Read the model definition and answer for the solid it produces. Units are mm, in the model's axes. A direction names the side the tool comes from. Coordinates: 2 decimals unless noted, no trailing zeros. Loops run counter-clockwise (first coordinate to the right, second up) from the corner with the lowest first, then second, coordinate; pieces in that order, holes last.
from build123d import *

# Parameters (mm, degrees)
F1_DEPTH = 7.5
F2_R     = 7.49999
F3_R     = 5
F4_DEPTH = 35.001
F5_R     = 5
F6_DEPTH = 27.501


# Not quite as in the source:
# - a fillet or chamfer is up to 0.001 mm smaller than in the source, because OpenCascade refuses the exact size


with BuildPart() as f1:
    # F0 (on Front) → F1 (new body, symmetric)
    with BuildSketch(Plane.XZ):
        with BuildLine():
            Line((7.5, 25), (-7.5, 25))
            Line((-7.5, 25), (-7.5, 20))
            Line((-7.5, 20), (7.5, 20))
            ThreePointArc((7.5, 20), (12.8033008589, 17.8033008589), (15, 12.5))
            Line((15, 12.5), (15, -10))
            Line((15, -10), (20, -10))
            Line((20, -10), (20, 12.5))
            ThreePointArc((20, 12.5), (16.3388347648, 21.3388347648), (7.5, 25))
        make_face()
    extrude(amount=F1_DEPTH, both=True)

    # F2 (radius 7.5 in the source; OpenCascade refuses exactly that, so slightly less here)
    f2_edges = [f1.edges().sort_by_distance(p)[0] for p in [
        (-7.5, -7.5, 22.5),
        (-7.5, 7.5, 22.5),
        (17.5, -7.5, -10),
        (17.5, 7.5, -10),
    ]]
    fillet(f2_edges, radius=F2_R)

    # F3 (on face) → F4 (cut, through all)
    with BuildSketch(Plane.XY.offset(25)):
        Circle(F3_R)
    extrude(amount=-F4_DEPTH, mode=Mode.SUBTRACT)

    # F5 (on face) → F6 (cut, through all)
    with BuildSketch(Plane.YZ.offset(20)):
        Circle(F5_R)
    extrude(amount=-F6_DEPTH, mode=Mode.SUBTRACT)


solid = f1.part
Item 1: A cutting plane is placed at A-A on z = 0. Determine the outline of the cut face in (x, y), then the cut area to 3 significant figures.
Numbers:
outline: (15, -7.5) - (20, -7.5) - (20, -5) - (15, -5) - close; (15, 5) - (20, 5) - (20, 7.5) - (15, 7.5) - close
area: 25.0 mm2
Item 2: A cutting plane is placed at C-C on x = -1. Determine the outline of the cut face in (y, z), then the cut area to 3 significant figures.
Numbers:
outline: (-7.43, 20) - (-4.9, 20) - (-4.9, 25) - (-7.43, 25) - close; (4.9, 20) - (7.43, 20) - (7.43, 25) - (4.9, 25) - close
area: 25.3 mm2
Item 3: Given pin 1 (7.5 mm diameter, centred on x = -2, y = -0.5, fed in from -Z); pin 2 (1 mm diameter, centred on y = -5.5, z = 17, fed in from +X); pin 3 (1 mm diameter, centred on x = 11, y = 0.5, fed in from +Z); pin 4 (3 mm diameter, centred on x = 3, y = 2.5, fed in from +Z), each flat-ended and moving along its own axis, determine where each tip first touches the part or whether it passes through.
Numbers:
pin 1: stops at z = 20
pin 2: stops at x = 19.34
pin 3: stops at z = 24.63
pin 4: stops at z = 25
Item 4: Determine the mould class of faces 3 (the face through (5, 2, 20)), 4 (the face through (17.54, -1.08, -4.88)), 5 (the face through (17.535, 5.245, -7.861)) for opening direction Y: released by +Y, released by -Y, zero draft, split by the parting line, or undercut.
Numbers:
face 3: zero draft
face 4: undercut
face 5: released by +Y
Item 5: Which of the six approach directions +Z, -Z, +X, -X, +Y, -Y give full straight-line access (tool end or side, diameter ignored) to faces 1 (the face through (20, 0, 6)), 2 (the face through (15, -3.4, 3.9))?
Numbers:
face 1: +Z, -Z, +X, +Y, -Y
face 2: -Z, -X, +Y, -Y
Item 6: Find the intervals of material crossed by line 1 along Y through (x, z) = (0, 21.4); line 2 along X through (y, z) = (5, -8); line 3 along Z through (x, y) = (18.2, 0), in increasing order.
Numbers:
line 1: y = -7.5 to -5, 5 to 7.5
line 2: x = 15 to 20
line 3: z = -10 to -5, 5 to 18.96
Item 7: A cutting plane is placed at B-B on y = -3.25. Determine the outline of the cut face in (x, z).
Numbers:
outline: (-6.76, 20) - (-3.8, 20) - (-3.8, 25) - (-6.76, 25) - close; (3.8, 20) - (7.5, 20) arc R7.5 cw to (15, 12.5) - (15, 3.8) - (20, 3.8) - (20, 12.5) arc R12.5 ccw to (7.5, 25) - (3.8, 25) - close; (15, -9.26) - (20, -9.26) - (20, -3.8) - (15, -3.8) - close
Item 8: A cutting plane is placed at D-D on y = 4. Determine the outline of the cut face in (x, z), then the cut area to 3 significant figures.
Numbers:
outline: (-6.34, 20) - (-3, 20) - (-3, 25) - (-6.34, 25) - close; (3, 20) - (7.5, 20) arc R7.5 cw to (15, 12.5) - (15, 3) - (20, 3) - (20, 12.5) arc R12.5 ccw to (7.5, 25) - (3, 25) - close; (15, -8.84) - (20, -8.84) - (20, -3) - (15, -3) - close
area: 194 mm2
